Build history of the part. All positions in model axes, mm. Face numbers are marked on the shaded views. A direction names the side the tool comes from. Coordinates: 2 decimals unless noted, no trailing zeros. Order: outer loops, then holes, each group sorted by start corner. A loop starts at its lowest first (then second) coordinate and runs counter-clockwise, first axis right, second up. Notation, with made-up numbers: (30.25, 2.5) - (52.25, 2.5) arc R21 cw to (52.25, 30.5) - close; hole circle Ø1 at (-8, 81.25). An arc over 180 degrees is marked (long way). Write each question's results on one line, items separated by ' | '. Start each with the question number.
from build123d import *

# Parameters (mm, degrees)
SKETCH2_W                                         = 80
SKETCH2_H                                         = 140
BOSS_EXTRUDE1_DEPTH                               = 50
SHELL1_T                                          = -5
SKETCH3_W                                         = 80
SKETCH3_H                                         = 140
SKETCH3_W_2                                       = 70
SKETCH3_H_2                                       = 130
BOSS_EXTRUDE2_DEPTH                               = 5
BOSS_EXTRUDE3_REACH                               = 99.596
CSK_FOR_0_FLAT_HEAD_MACHINE_SCREW_100_D           = 1.6129
CSK_FOR_0_FLAT_HEAD_MACHINE_SCREW_100_DEPTH       = 10
CSK_FOR_0_FLAT_HEAD_MACHINE_SCREW_100_CSINK_D     = 3.0226
CSK_FOR_0_FLAT_HEAD_MACHINE_SCREW_100_CSINK_ANGLE = 100
CSK_FOR_0_FLAT_HEAD_MACHINE_SCREW_100_TIP         = 0.484564046
FILLET1_R                                         = 10
FILLET2_R                                         = 2.5


with BuildPart() as part:
    # Sketch2 → Boss-Extrude1 (new body)
    with BuildSketch(Plane(origin=(0, 0, 0), x_dir=(1, 0, 0), z_dir=(0, 1, 0))):
        Rectangle(SKETCH2_W, SKETCH2_H)
    extrude(amount=BOSS_EXTRUDE1_DEPTH)

    # Shell1
    shell1_openings = [part.faces().sort_by_distance(p)[0] for p in [
        (0, 50, 0),
    ]]
    offset(amount=SHELL1_T, openings=shell1_openings, kind=Kind.INTERSECTION)

    # Sketch3 → Boss-Extrude2 (add)
    with BuildSketch(Plane(origin=(0, 50, 0), x_dir=(1, 0, 0), z_dir=(0, 1, 0))):
        Rectangle(SKETCH3_W, SKETCH3_H)
        Rectangle(SKETCH3_W_2, SKETCH3_H_2, mode=Mode.SUBTRACT)
    extrude(amount=BOSS_EXTRUDE2_DEPTH)

    # Sketch4 → Boss-Extrude3 (add, up to next)
    with BuildSketch(Plane(origin=(0, 55, 0), x_dir=(1, 0, 0), z_dir=(0, 1, 0)), mode=Mode.PRIVATE) as boss_extrude3_sk1:
        with BuildLine():
            Line((-35, -65), (-35, -55))
            Line((-35, -55), (-30, -55))
            ThreePointArc((-30, -55), (-26.464466094, -56.464466094), (-25, -60))
            Line((-25, -60), (-25, -65))
            Line((-25, -65), (-35, -65))
        make_face()
    boss_extrude3_tool1 = extrude(boss_extrude3_sk1.sketch, amount=-BOSS_EXTRUDE3_REACH, mode=Mode.PRIVATE) - part.part
    # Sketch4 → Boss-Extrude3 (add, up to next)
    with BuildSketch(Plane(origin=(0, 55, 0), x_dir=(1, 0, 0), z_dir=(0, 1, 0)), mode=Mode.PRIVATE) as boss_extrude3_sk2:
        with BuildLine():
            Line((30, -55), (35, -55))
            Line((35, -55), (35, -65))
            Line((35, -65), (25, -65))
            Line((25, -65), (25, -60))
            ThreePointArc((25, -60), (26.464466094, -56.464466094), (30, -55))
        make_face()
    boss_extrude3_tool2 = extrude(boss_extrude3_sk2.sketch, amount=-BOSS_EXTRUDE3_REACH, mode=Mode.PRIVATE) - part.part
    # Sketch4 → Boss-Extrude3 (add, up to next)
    with BuildSketch(Plane(origin=(0, 55, 0), x_dir=(1, 0, 0), z_dir=(0, 1, 0)), mode=Mode.PRIVATE) as boss_extrude3_sk3:
        with BuildLine():
            Line((25, 60), (25, 65))
            Line((25, 65), (35, 65))
            Line((35, 65), (35, 55))
            Line((35, 55), (30, 55))
            ThreePointArc((30, 55), (26.464466094, 56.464466094), (25, 60))
        make_face()
    boss_extrude3_tool3 = extrude(boss_extrude3_sk3.sketch, amount=-BOSS_EXTRUDE3_REACH, mode=Mode.PRIVATE) - part.part
    # Sketch4 → Boss-Extrude3 (add, up to next)
    with BuildSketch(Plane(origin=(0, 55, 0), x_dir=(1, 0, 0), z_dir=(0, 1, 0)), mode=Mode.PRIVATE) as boss_extrude3_sk4:
        with BuildLine():
            Line((-30, 55), (-35, 55))
            Line((-35, 55), (-35, 65))
            Line((-35, 65), (-25, 65))
            Line((-25, 65), (-25, 60))
            ThreePointArc((-25, 60), (-26.464466094, 56.464466094), (-30, 55))
        make_face()
    boss_extrude3_tool4 = extrude(boss_extrude3_sk4.sketch, amount=-BOSS_EXTRUDE3_REACH, mode=Mode.PRIVATE) - part.part
    add(boss_extrude3_tool1.solids().sort_by_distance((-30.220144, 55, 60.220144))[0])
    add(boss_extrude3_tool2.solids().sort_by_distance((30.220144, 55, 60.220144))[0])
    add(boss_extrude3_tool3.solids().sort_by_distance((30.220144, 55, -60.220144))[0])
    add(boss_extrude3_tool4.solids().sort_by_distance((-30.220144, 55, -60.220144))[0])

    # CSK for #0 Flat Head Machine Screw (100)1
    with Locations(Plane(origin=(0, 55, 0), x_dir=(1, 0, 0), z_dir=(0, 1, 0))):
        with Locations((-30.216332876, -59.957909435), (29.772350977, -59.957909435), (29.772350977, 60.028429813), (-30.216332876, 60.028429813)):
            CounterSinkHole(CSK_FOR_0_FLAT_HEAD_MACHINE_SCREW_100_D / 2, CSK_FOR_0_FLAT_HEAD_MACHINE_SCREW_100_CSINK_D / 2, depth=CSK_FOR_0_FLAT_HEAD_MACHINE_SCREW_100_DEPTH, counter_sink_angle=CSK_FOR_0_FLAT_HEAD_MACHINE_SCREW_100_CSINK_ANGLE)
            with Locations((0, 0, -(CSK_FOR_0_FLAT_HEAD_MACHINE_SCREW_100_DEPTH + CSK_FOR_0_FLAT_HEAD_MACHINE_SCREW_100_TIP / 2))):  # 118° drill point
                Cone(0, CSK_FOR_0_FLAT_HEAD_MACHINE_SCREW_100_D / 2, CSK_FOR_0_FLAT_HEAD_MACHINE_SCREW_100_TIP, mode=Mode.SUBTRACT)

    # Fillet1
    fillet1_edges = [part.edges().sort_by_distance(p)[0] for p in [
        (40, 27.5, 70),
        (-40, 27.5, 70),
        (-40, 27.5, -70),
        (40, 27.5, -70),
    ]]
    fillet(fillet1_edges, radius=FILLET1_R)

    # Fillet2
    fillet2_edges = [part.edges().sort_by_distance(p)[0] for p in [
        (-40, 0, 0),
        (40, 0, 0),
        (0, 0, 70),
        (0, 0, -70),
        (37.071067812, 0, 67.071067812),
        (-37.071067812, 0, 67.071067812),
        (37.071067812, 0, -67.071067812),
        (-37.071067812, 0, -67.071067812),
    ]]
    fillet(fillet2_edges, radius=FILLET2_R)


solid = part.part
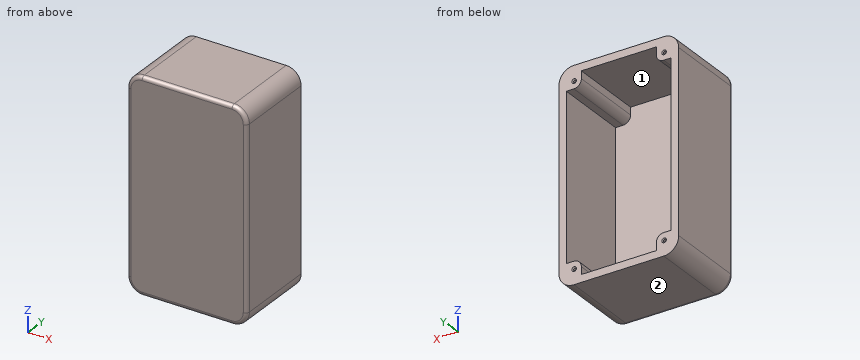
Item 1: Slice it at A-A (y = 37). Write the cut outline in (x, z).
Item 2: Which spindle directions (+Z, -Z, +X, -X, +Y, -Y) get a long thin tool onto all of the face, cutting with end or side? Do the marked faces 1 and 2. Say none if no direction does.
Item 3: Slice it at C-C (x = 14). Write the cut outline in (y, z).
Item 4: Flat gauge pins, fed straight in: P1, Ø2.5, axis at x = 29.77, z = 59.96, coming from the +Y side; P2, Ø10, axis at x = -3.5, z = -49, coming from the +Y side; P3, Ø1.5, axis at x = 31.5, y = 18, coming from the -Z side. Where does each tip first touch, or does it go through?
Item 5: Probe probe 1 along Z at (x, y) = (-11, 18); probe 2 along X at (y, z) = (44.5, -3); probe 3 along Y at (x, z) = (8, 15). List the from-to ranges inside material, lowest first.
Item 6: Slice it at B-B (z = -51.5). Write the cut outline in (x, y), then the cut area to 3 significant figures.
Resolved:
1) outline: (-40, -60) arc R10 ccw to (-30, -70) - (30, -70) arc R10 ccw to (40, -60) - (40, 60) arc R10 ccw to (30, 70) - (-30, 70) arc R10 ccw to (-40, 60) - close; hole (-35, -55) - (-30, -55) arc R5 cw to (-25, -60) - (-25, -65) - (25, -65) - (25, -60) arc R5 cw to (30, -55) - (35, -55) - (35, 55) - (30, 55) arc R5 cw to (25, 60) - (25, 65) - (-25, 65) - (-25, 60) arc R5 cw to (-30, 55) - (-35, 55) - close
2) face 1: +Y | face 2: -Z, +X, -X, +Y, -Y
3) outline: (0, -67.5) arc R2.5 ccw to (2.5, -70) - (55, -70) - (55, -65) - (5, -65) - (5, 65) - (55, 65) - (55, 70) - (2.5, 70) arc R2.5 ccw to (0, 67.5) - close
4) P1: y = 54.78 | P2: y = 5 | P3: z = -69.97
5) probe 1: -70 to -65, 65 to 70 | probe 2: -40 to -35, 35 to 40 | probe 3: 0 to 5
6) outline: (-40, 2.5) arc R2.5 ccw to (-37.5, 0) - (37.5, 0) arc R2.5 ccw to (40, 2.5) - (40, 55) - (35, 55) - (35, 5) - (-35, 5) - (-35, 55) - (-40, 55) - close | area: 897 mm^2
